```python
from build123d import *

# Parameters (mm, degrees)
PAD024_DEPTH    = 34.5
POCKET023_DEPTH = 31.5
SKETCH055_R     = 2.05
SKETCH055_R_2   = 2
POCKET024_DEPTH = 6.2
SKETCH057_R     = 3
SKETCH057_R_2   = 5
SKETCH057_R_3   = 3.5
PAD025_DEPTH    = 17.5
SKETCH058_R     = 2.55
SKETCH058_R_2   = 2.05
POCKET026_DEPTH = 6.2
FILLET001_R     = 3
SKETCH059_W     = 20
SKETCH059_H     = 10
POCKET027_DEPTH = 5
SKETCH060_W     = 20
SKETCH060_H     = 10
POCKET028_DEPTH = 5


with BuildPart() as part:
    # Sketch052 → Pad024 (new body)
    with BuildSketch(Plane.XZ):
        with BuildLine():
            ThreePointArc((-0.5, 13.5), (2.428932, 6.428932), (9.5, 3.5))
            Line((9.5, 3.5), (192.51, 3.5))
            ThreePointArc((192.51, 3.5), (199.581068, 6.428932), (202.51, 13.5))
            Line((202.51, 13.5), (202.51, 109.54))
            ThreePointArc((202.51, 109.54), (199.581068, 116.611068), (192.51, 119.54))
            Line((192.51, 119.54), (97.391395, 119.54))
            ThreePointArc((97.391395, 119.54), (96.36955, 119.672723), (95.415517, 120.062083))
            Line((95.415517, 120.062083), (67.291034, 136.040187))
            ThreePointArc((67.291034, 136.040187), (65.859984, 136.624227), (64.327218, 136.823311))
            Line((64.327218, 136.823311), (35.377399, 136.823311))
            ThreePointArc((35.377399, 136.823311), (30.31762, 135.448776), (26.64881, 131.703038))
            Line((26.64881, 131.703038), (2.447131, 88.412394))
            ThreePointArc((2.447131, 88.412394), (0.24888, 82.945607), (-0.5, 77.101188))
            Line((-0.5, 77.101188), (-0.5, 13.5))
        make_face()
    extrude(amount=PAD024_DEPTH)

    # Sketch054 (on Face16 of Pad024) → Pocket023 (cut)
    with BuildSketch(Plane.XZ.offset(34.5)):
        with BuildLine():
            ThreePointArc((5.5, 15.5), (8.428932, 8.428932), (15.5, 5.5))
            Line((15.5, 5.5), (186.51, 5.5))
            ThreePointArc((186.51, 5.5), (193.581068, 8.428932), (196.51, 15.5))
            Line((196.51, 15.5), (196.51, 107.54))
            ThreePointArc((196.51, 107.54), (193.581068, 114.611068), (186.51, 117.54))
            Line((186.51, 117.54), (96.852925, 117.54))
            ThreePointArc((96.852925, 117.54), (95.816521, 117.676599), (94.850903, 118.077066))
            Line((94.850903, 118.077066), (67.278075, 134.017712))
            ThreePointArc((67.278075, 134.017712), (65.829649, 134.618413), (64.275043, 134.823311))
            Line((64.275043, 134.823311), (41.153265, 134.823311))
            ThreePointArc((41.153265, 134.823311), (36.151908, 133.482781), (32.491444, 129.820596))
            Line((32.491444, 129.820596), (8.601898, 88.412711))
            ThreePointArc((8.601898, 88.412711), (6.288899, 82.824921), (5.5, 76.829005))
            Line((5.5, 76.829005), (5.5, 15.5))
        make_face()
    extrude(amount=-POCKET023_DEPTH, mode=Mode.SUBTRACT)

    # Sketch055 (on Face5 of Pocket023) → Pocket024 (cut)
    with BuildSketch(Plane.XZ.offset(34.5)):
        with Locations((199.51, 21.5)):
            Circle(SKETCH055_R)
        with Locations((199.51, 101.5)):
            Circle(SKETCH055_R)
        with Locations((199.51, 41.5)):
            Circle(SKETCH055_R)
        with Locations((199.51, 81.5)):
            Circle(SKETCH055_R)
        with Locations((199.51, 61.5)):
            Circle(SKETCH055_R)
        with Locations((2.5, 25.5)):
            Circle(SKETCH055_R)
        with Locations((2.5, 45.5)):
            Circle(SKETCH055_R)
        with Locations((2.5, 65.5)):
            Circle(SKETCH055_R)
        with Locations((7.984524, 92.743621)):
            Circle(SKETCH055_R_2)
        with Locations((17.909674, 110.107129)):
            Circle(SKETCH055_R_2)
        with Locations((27.944341, 127.407576)):
            Circle(SKETCH055_R_2)
    extrude(amount=-POCKET024_DEPTH, mode=Mode.SUBTRACT)

    # Sketch057 (on Face51 of Pocket024) → Pad025 (join)
    with BuildSketch(Plane.XZ.offset(3)):
        with Locations((74.17, 12.74)):
            Circle(SKETCH057_R)
        with Locations((64.332465, 127.473311)):
            Circle(SKETCH057_R_2)
        with Locations((105.902925, 108.54)):
            Circle(SKETCH057_R)
        with Locations((145.13, 13)):
            Circle(SKETCH057_R_3)
        with Locations((188.34, 14.18)):
            Circle(SKETCH057_R_2)
        with Locations((185.61, 111.04)):
            Circle(SKETCH057_R_2)
        with Locations((14.14, 13.53)):
            Circle(SKETCH057_R_2)
    extrude(amount=PAD025_DEPTH)

    # Sketch058 (on Face63 of Pad025) → Pocket026 (cut)
    with BuildSketch(Plane.XZ.offset(20.5)):
        with Locations((64.332465, 127.473311)):
            Circle(SKETCH058_R)
        with Locations((105.902925, 108.54)):
            Circle(SKETCH058_R_2)
        with Locations((14.14, 13.53)):
            Circle(SKETCH058_R)
        with Locations((74.17, 12.74)):
            Circle(SKETCH058_R_2)
        with Locations((145.13, 13)):
            Circle(SKETCH058_R_2)
        with Locations((188.34, 14.18)):
            Circle(SKETCH058_R)
        with Locations((185.61, 111.04)):
            Circle(SKETCH058_R)
    extrude(amount=-POCKET026_DEPTH, mode=Mode.SUBTRACT)

    # Fillet001
    fillet001_edges = [part.edges().sort_by_distance(p)[0] for p in [
        (2.428932, 0, 6.428932),
        (101.005, 0, 3.5),
        (199.581068, 0, 6.428932),
        (202.51, 0, 61.52),
        (199.581068, 0, 116.611068),
        (144.950697, 0, 119.54),
        (96.36955, 0, 119.672723),
        (81.353275, 0, 128.051135),
        (65.859984, 0, 136.624227),
        (49.852308, 0, 136.823311),
        (30.31762, 0, 135.448776),
        (14.54797, 0, 110.057716),
        (0.24888, 0, 82.945607),
        (-0.5, 0, 45.300594),
    ]]
    fillet(fillet001_edges, radius=FILLET001_R)

    # Sketch059 (on Face16 of Fillet001) → Pocket027 (cut)
    with BuildSketch(Plane(origin=(0, 0, 119.54), x_dir=(-1, 0, 0), z_dir=(0, 0, 1))):
        with Locations((-107.391395, 29.5)):
            Rectangle(SKETCH059_W, SKETCH059_H)
    extrude(amount=-POCKET027_DEPTH, mode=Mode.SUBTRACT)

    # Sketch060 (on Face5 of Pocket027) → Pocket028 (cut)
    with BuildSketch(Plane(origin=(0, 0, 3.5), x_dir=(1, 0, 0), z_dir=(0, 0, -1))):
        with Locations((107.391395, 29.5)):
            Rectangle(SKETCH060_W, SKETCH060_H)
    extrude(amount=-POCKET028_DEPTH, mode=Mode.SUBTRACT)


with BuildPart() as part_1:
    # Body006 placement: moved
    add(part.part.moved(Location((0, 20.5, 0))))


solid = part_1.part
```
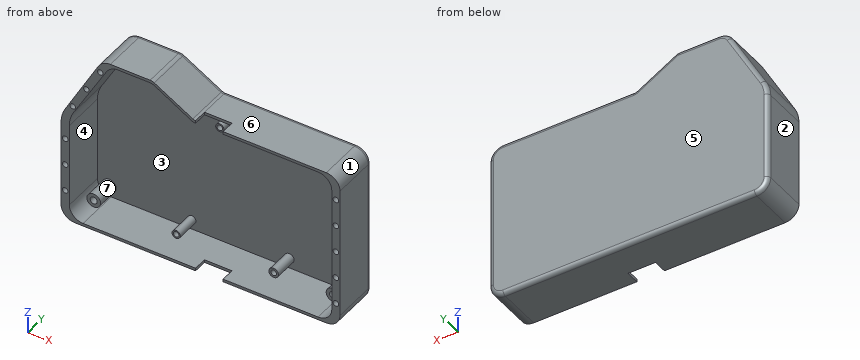
For this review, take the finished solid that the model builds, in its own axes (mm). Face numbers are marked on the shaded views. A direction names the side the tool comes from. Round coordinates to 2 decimals unless told otherwise and drop trailing zeros. Write each loop counter-clockwise with the first axis right and the second up, starting at its lowest first coordinate (ties: lowest second). Pieces come first, ordered by that corner, then holes. Notation, with made-up numbers: M 29,39.5 L 72,39.5 A9 ccw 72,55.5 Z; hole C 82,10 d1. An arc over 180 degrees is marked long. One line per item, written item: value. Start each with the question number.
(1) Wall thickness on line 1 (Z direction, x = 148, y = 2); line 2 (X direction, y = 4, z = 111); line 3 (Z direction, x = 152, y = -13): over which ranges is each line inside the solid? List them lowest first.
(2) We need section B-B (z = 37). Give the boundary of the cut face in (x, y).
(3) The part is to be moulded in two halves that separate along X. For the marked faces 1, 2, 3 and 4, say which applies: released by +X, released by -X, zero draft, split by the parting line, or undercut.
(4) Machinability: for the marked faces 5, 6 and 7, which of the approach directions +Z, -Z, +X, -X, +Y, -Y give a long, thin tool a straight path to every point of the face, cutting with its end or side? Answer none if there is none.
(5) Insertion check: pin 1 (1.8 mm diameter, centred on x = 105, z = 108.5, fed in from -Y); pin 2 (3 mm diameter, centred on x = 70, y = 9.5, fed in from +Z); pin 3 (1.2 mm diameter, centred on x = 2, z = 26, fed in from -Y); pin 4 (4.5 mm diameter, centred on x = 199, z = 21.5, fed in from -Y). Each pin has a flat end and moves straight along its axis. Give the tip position at first contact, or say it passes through.
(6) We need section C-C (y = 15.5). Count the separate pieces of the cut face and the enclosed holes in it, and give its area (3 significant figures).
(7) We need section A-A (x = 156.5). Give the boundary of the cut face in (y, z).
Result:
1. line 1: 3.5 to 5.5, 11 to 15, 117.54 to 119.54
1. line 2: 15.07 to 21.63, 104.19 to 107.62, 180.61 to 183.06, 188.16 to 190.61, 195.89 to 202.4
1. line 3: 3.5 to 5.5, 117.54 to 119.54
2. outline: M -0.5,-14 L 5.5,-14 L 5.5,17.5 L 196.51,17.5 L 196.51,-14 L 202.51,-14 L 202.51,17.5 A3 ccw 199.51,20.5 L 2.5,20.5 A3 ccw -0.5,17.5 Z
3. face 1: released by +X
3. face 2: released by -X
3. face 3: undercut
3. face 4: undercut
4. face 5: +Z, -Z, +X, -X, +Y
4. face 6: +Z, +X, +Y, -Y
4. face 7: -Y
5. pin 1: y = 6.2
5. pin 2: z = 135.35
5. pin 3: y = -7.8
5. pin 4: y = -14
6. separate pieces: 8
6. enclosed holes: 1
6. area: 2,640 mm²
7. outline: M -14,3.5 L 17.5,3.5 A3 ccw 20.5,6.5 L 20.5,116.54 A3 ccw 17.5,119.54 L -14,119.54 L -14,117.54 L 17.5,117.54 L 17.5,5.5 L -14,5.5 Z
